Work out the finished part from the listing and answer in its coordinate system (mm). Face numbers are marked on the shaded views. A direction names the side the tool comes from. Round coordinates to 2 decimals unless told otherwise and drop trailing zeros. Order: outer loops, then holes, each group sorted by start corner. A loop starts at its lowest first (then second) coordinate and runs counter-clockwise, first axis right, second up. Notation, with made-up numbers: (1.5, 54.25) - (17.5, 54.25) arc R23 ccw to (17.5, 62.25) - close; hole circle Ø2 at (24.5, 34). An arc over 180 degrees is marked (long way). Answer in a Markdown table with one row per item.
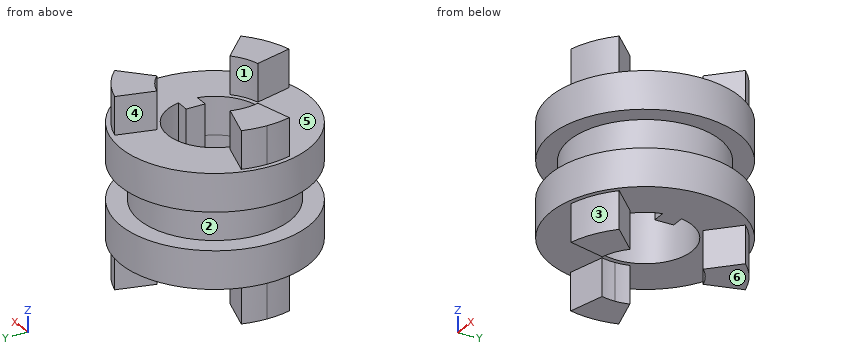
from build123d import *

# Parameters (mm, degrees)
SKETCH1_R           = 10
SKETCH1_R_2         = 5
BOSS_EXTRUDE2_DEPTH = 4
BOSS_EXTRUDE3_DEPTH = 4
SKETCH3_W           = 3
SKETCH3_H           = 2
BOSS_EXTRUDE4_DEPTH = 4
BOSS_EXTRUDE5_START = 4
SKETCH4_R           = 8
BOSS_EXTRUDE5_DEPTH = 4
BOSS_EXTRUDE6_START = 4
SKETCH5_R           = 10
BOSS_EXTRUDE6_DEPTH = 4
BOSS_EXTRUDE7_START = 4
BOSS_EXTRUDE7_DEPTH = 4
BOSS_EXTRUDE8_DEPTH = 10


with BuildPart() as part:
    # Sketch1 → Boss-Extrude2 (new body)
    with BuildSketch(Plane.XY):
        Circle(SKETCH1_R)
        Circle(SKETCH1_R_2, mode=Mode.SUBTRACT)
    extrude(amount=BOSS_EXTRUDE2_DEPTH)

    # Sketch2 → Boss-Extrude3 (add)
    with BuildSketch(Plane.XY.offset(4)):
        with BuildLine():
            ThreePointArc((-5.5, 0), (-5.449982192, 0.74006358), (-5.300838508, 1.466666667))
            Line((-5.300838508, 1.466666667), (-9.155993787, 2.533333333))
            ThreePointArc((-9.155993787, 2.533333333), (-9.413605605, 1.278291639), (-9.5, 0))
            ThreePointArc((-9.5, 0), (-9.413605605, -1.278291639), (-9.155993787, -2.533333333))
            Line((-9.155993787, -2.533333333), (-5.300838508, -1.466666667))
            ThreePointArc((-5.300838508, -1.466666667), (-5.449982192, -0.74006358), (-5.5, 0))
        make_face()
        with BuildLine():
            ThreePointArc((3.920589846, -3.857327476), (2.75, -4.763139721), (1.380248662, -5.323994143))
            Line((1.380248662, -5.323994143), (2.38406587, -9.195989883))
            ThreePointArc((2.38406587, -9.195989883), (4.75, -8.227241336), (6.771927916, -6.66265655))
            Line((6.771927916, -6.66265655), (3.920589846, -3.857327476))
        make_face()
        with BuildLine():
            Line((2.38406587, 9.195989883), (1.380248662, 5.323994143))
            ThreePointArc((1.380248662, 5.323994143), (2.75, 4.763139721), (3.920589846, 3.857327476))
            Line((3.920589846, 3.857327476), (6.771927916, 6.66265655))
            ThreePointArc((6.771927916, 6.66265655), (4.75, 8.227241336), (2.38406587, 9.195989883))
        make_face()
    extrude(amount=BOSS_EXTRUDE3_DEPTH)

    # Sketch3 → Boss-Extrude4 (add)
    with BuildSketch(Plane(origin=(0, 0, 0), x_dir=(-1, 0, 0), z_dir=(0, 0, -1))):
        with Locations((-5, 0)):
            Rectangle(SKETCH3_W, SKETCH3_H)
    extrude(amount=-BOSS_EXTRUDE4_DEPTH)

    # Sketch4 → Boss-Extrude5 (add)
    with BuildSketch(Plane(origin=(0, 0, 0), x_dir=(-1, 0, 0), z_dir=(0, 0, -1)).offset(BOSS_EXTRUDE5_START)):
        Circle(SKETCH4_R)
        with BuildLine():
            Line((-4.974937186, 0.5), (-3.5, 0.5))
            Line((-3.5, 0.5), (-3.5, -1))
            Line((-3.5, -1), (-4.898979486, -1))
            ThreePointArc((-4.898979486, -1), (4.993601667, 0.252868331), (-4.974937186, 0.5))
        make_face(mode=Mode.SUBTRACT)
    extrude(amount=-BOSS_EXTRUDE5_DEPTH)

    # Sketch5 → Boss-Extrude6 (add)
    with BuildSketch(Plane(origin=(0, 0, -4), x_dir=(-1, 0, 0), z_dir=(0, 0, -1)).offset(BOSS_EXTRUDE6_START)):
        with Locations(Location((0, 0, 0), (0, 0, 180))):
            Circle(SKETCH5_R)
        with BuildLine():
            Line((-4.974937186, 0.5), (-3.5, 0.5))
            Line((-3.5, 0.5), (-3.5, -1))
            Line((-3.5, -1), (-4.898979486, -1))
            ThreePointArc((-4.898979486, -1), (4.993601667, 0.252868331), (-4.974937186, 0.5))
        make_face(mode=Mode.SUBTRACT)
    extrude(amount=-BOSS_EXTRUDE6_DEPTH)

    # Sketch6 → Boss-Extrude7 (add)
    with BuildSketch(Plane(origin=(0, 0, -8), x_dir=(-1, 0, 0), z_dir=(0, 0, -1)).offset(BOSS_EXTRUDE7_START)):
        with BuildLine():
            ThreePointArc((-3.920589846, 3.857327476), (-2.75, 4.763139721), (-1.380248662, 5.323994143))
            Line((-1.380248662, 5.323994143), (-2.38406587, 9.195989883))
            ThreePointArc((-2.38406587, 9.195989883), (-4.75, 8.227241336), (-6.771927916, 6.66265655))
            Line((-6.771927916, 6.66265655), (-3.920589846, 3.857327476))
        make_face()
        with BuildLine():
            ThreePointArc((-1.380248662, -5.323994143), (-2.75, -4.763139721), (-3.920589846, -3.857327476))
            Line((-3.920589846, -3.857327476), (-6.771927916, -6.66265655))
            ThreePointArc((-6.771927916, -6.66265655), (-4.75, -8.227241336), (-2.38406587, -9.195989883))
            Line((-2.38406587, -9.195989883), (-1.380248662, -5.323994143))
        make_face()
        with BuildLine():
            Line((9.155993787, 2.533333333), (5.300838508, 1.466666667))
            ThreePointArc((5.300838508, 1.466666667), (5.449982192, 0.74006358), (5.5, 0))
            ThreePointArc((5.5, 0), (5.449982192, -0.74006358), (5.300838508, -1.466666667))
            Line((5.300838508, -1.466666667), (9.155993787, -2.533333333))
            ThreePointArc((9.155993787, -2.533333333), (9.413605605, -1.278291639), (9.5, 0))
            ThreePointArc((9.5, 0), (9.413605605, 1.278291639), (9.155993787, 2.533333333))
        make_face()
    extrude(amount=-BOSS_EXTRUDE7_DEPTH)

    # Sketch10 → Boss-Extrude8 (add)
    with BuildSketch(Plane(origin=(0, 0, -8), x_dir=(-1, 0, 0), z_dir=(0, 0, -1))):
        with BuildLine():
            Line((-3.5, 1), (-4.898979486, 1))
            ThreePointArc((-4.898979486, 1), (-4.943284091, 0.75096098), (-4.974937186, 0.5))
            Line((-4.974937186, 0.5), (-3.5, 0.5))
            Line((-3.5, 0.5), (-3.5, 1))
        make_face()
    extrude(amount=-BOSS_EXTRUDE8_DEPTH)


solid = part.part
1) The mould has two halves that part along Y. Classify the marked faces 4, 5 and 6: released by +Y, released by -Y, zero draft, split by the parting line, or undercut.
Filled in:
| item | result |
|---|---|
| face 4 | released by +Y |
| face 5 | undercut |
| face 6 | zero draft |
2) Find section D-D, the plane z = -7. Give the vertices of the cut face in (x, y), then the cut area to 3 significant figures.
Filled in:
| item | result |
|---|---|
| outline | circle Ø20 at (0, 0); hole (3.5, -1) - (3.5, 1) - (4.9, 1) arc R5 ccw (long way) to (4.9, -1) - close |
| area | 239 mm^2 |
3) Which of the six approach directions +Z, -Z, +X, -X, +Y, -Y give full straight-line access (tool end or side, diameter ignored) to the marked faces 1, 2 and 3?
Filled in:
| item | result |
|---|---|
| face 1 | +Z, -X |
| face 2 | none |
| face 3 | -Z, +X, -Y |
4) Find section A-A, the plane z = 5.25. Give the vertices of the cut face in (x, y), then the cut area to 3 significant figures.
Filled in:
| item | result |
|---|---|
| outline | (-9.16, -2.53) - (-5.3, -1.47) arc R5.5 cw to (-5.3, 1.47) - (-9.16, 2.53) arc R9.5 ccw to start; (1.38, -5.32) - (2.38, -9.2) arc R9.5 ccw to (6.77, -6.66) - (3.92, -3.86) arc R5.5 cw to start; (1.38, 5.32) arc R5.5 cw to (3.92, 3.86) - (6.77, 6.66) arc R9.5 ccw to (2.38, 9.2) - close |
| area | 48.6 mm^2 |
5) Find section B-B, the plane x = 0. Give the vertices of the cut face in (y, z).
Filled in:
| item | result |
|---|---|
| outline | (-10, -8) - (-5, -8) - (-5, 4) - (-10, 4) - (-10, 0) - (-8, 0) - (-8, -4) - (-10, -4) - close; (5, -8) - (10, -8) - (10, -4) - (8, -4) - (8, 0) - (10, 0) - (10, 4) - (5, 4) - close |
6) Each of these flat-tipped pins is pushed along its axis until it touches: pin 1 (1.5 mm diameter, centred on x = 4.5, z = -2.5, fed in from -Y); pin 2 (3 mm diameter, centred on x = -7.5, y = -7, fed in from +Z); pin 3 (0.7 mm diameter, centred on x = 4, z = -2, fed in from +Y). Where does it stop, or does it pass through?
Filled in:
| item | result |
|---|---|
| pin 1 | stops at y = -7.07 |
| pin 2 | stops at z = 4 |
| pin 3 | stops at y = 7.12 |
7) Find the intervals of material crossed by probe 1 along Y at (x, z) = (0, -2); probe 2 along Y at (x, z) = (0, 2.7); probe 3 along Z at (x, y) = (9.25, 2.25), in increasing order. Write a range as from..to.
Filled in:
| item | result |
|---|---|
| probe 1 | y = -8..-5, 5..8 |
| probe 2 | y = -10..-5, 5..10 |
| probe 3 | z = -8..-4, 0..4 |
8) Find section C-C, the plane y = -2. Give the vertices of the cut face in (x, z).
Filled in:
| item | result |
|---|---|
| outline | (-9.8, -8) - (-9.29, -8) - (-9.29, -12) - (-7.23, -12) - (-7.23, -8) - (-4.58, -8) - (-4.58, 4) - (-7.23, 4) - (-7.23, 8) - (-9.29, 8) - (-9.29, 4) - (-9.8, 4) - (-9.8, 0) - (-7.75, 0) - (-7.75, -4) - (-9.8, -4) - close; (4.58, -8) - (9.8, -8) - (9.8, -4) - (7.75, -4) - (7.75, 0) - (9.8, 0) - (9.8, 4) - (4.58, 4) - close |
